from build123d import *

# Parameters (mm, degrees)
SKETCH1_R           = 2
BOSS_EXTRUDE1_DEPTH = 2.5
SKETCH2_W           = 35
SKETCH2_H           = 4
BOSS_EXTRUDE2_DEPTH = 35
CUT_EXTRUDE1_REACH  = 6
SKETCH3_R           = 1.5
SKETCH3_R_2         = 7.75


with BuildPart() as part:
    # Sketch1 → Boss-Extrude1 (new body, symmetric)
    with BuildSketch(Plane(origin=(0, 0, 0), x_dir=(1, 0, 0), z_dir=(0, 1, 0))):
        Polygon((17.5, 45), (-5.5, 45), (-5.5, -10), (-17.5, -10), (-17.5, -45), (17.5, -45), align=None)
        with Locations((-11.75, -20)):
            Circle(SKETCH1_R, mode=Mode.SUBTRACT)
        with BuildLine():
            ThreePointArc((13.75, -20), (11.75, -22), (9.75, -20))
            ThreePointArc((9.75, -20), (11.75, -18), (13.75, -20))
        make_face(mode=Mode.SUBTRACT)
        with Locations((11.75, -1.5)):
            Circle(SKETCH1_R, mode=Mode.SUBTRACT)
    extrude(amount=BOSS_EXTRUDE1_DEPTH, both=True)

    # Sketch2 → Boss-Extrude2 (add)
    with BuildSketch(Plane(origin=(0, 2.5, 0), x_dir=(1, 0, 0), z_dir=(0, 1, 0))):
        with Locations((0, -43)):
            Rectangle(SKETCH2_W, SKETCH2_H)
    extrude(amount=BOSS_EXTRUDE2_DEPTH)

    # Sketch3 → Cut-Extrude1 (cut, up to next)
    with BuildSketch(Plane(origin=(0, 0, 41), x_dir=(-1, 0, 0), z_dir=(0, 0, -1)), mode=Mode.PRIVATE) as cut_extrude1_sk1:
        with Locations((-12.2, 20)):
            Circle(SKETCH3_R)
    cut_extrude1_tool1 = extrude(cut_extrude1_sk1.sketch, amount=-CUT_EXTRUDE1_REACH, mode=Mode.PRIVATE) & part.part
    add(cut_extrude1_tool1.solids().sort_by_distance((12.2, 20, 41))[0], mode=Mode.SUBTRACT)
    # Sketch3 → Cut-Extrude1 (cut, up to next)
    with BuildSketch(Plane(origin=(0, 0, 41), x_dir=(-1, 0, 0), z_dir=(0, 0, -1)), mode=Mode.PRIVATE) as cut_extrude1_sk2:
        with Locations((0, 32.2)):
            Circle(SKETCH3_R)
    cut_extrude1_tool2 = extrude(cut_extrude1_sk2.sketch, amount=-CUT_EXTRUDE1_REACH, mode=Mode.PRIVATE) & part.part
    add(cut_extrude1_tool2.solids().sort_by_distance((0, 32.2, 41))[0], mode=Mode.SUBTRACT)
    # Sketch3 → Cut-Extrude1 (cut, up to next)
    with BuildSketch(Plane(origin=(0, 0, 41), x_dir=(-1, 0, 0), z_dir=(0, 0, -1)), mode=Mode.PRIVATE) as cut_extrude1_sk3:
        with Locations((12.2, 20)):
            Circle(SKETCH3_R)
    cut_extrude1_tool3 = extrude(cut_extrude1_sk3.sketch, amount=-CUT_EXTRUDE1_REACH, mode=Mode.PRIVATE) & part.part
    add(cut_extrude1_tool3.solids().sort_by_distance((-12.2, 20, 41))[0], mode=Mode.SUBTRACT)
    # Sketch3 → Cut-Extrude1 (cut, up to next)
    with BuildSketch(Plane(origin=(0, 0, 41), x_dir=(-1, 0, 0), z_dir=(0, 0, -1)), mode=Mode.PRIVATE) as cut_extrude1_sk4:
        with Locations((0, 20)):
            Circle(SKETCH3_R_2)
    cut_extrude1_tool4 = extrude(cut_extrude1_sk4.sketch, amount=-CUT_EXTRUDE1_REACH, mode=Mode.PRIVATE) & part.part
    add(cut_extrude1_tool4.solids().sort_by_distance((0, 20, 41))[0], mode=Mode.SUBTRACT)
    # Sketch3 → Cut-Extrude1 (cut, up to next)
    with BuildSketch(Plane(origin=(0, 0, 41), x_dir=(-1, 0, 0), z_dir=(0, 0, -1)), mode=Mode.PRIVATE) as cut_extrude1_sk5:
        with Locations((0, 7.8)):
            Circle(SKETCH3_R)
    cut_extrude1_tool5 = extrude(cut_extrude1_sk5.sketch, amount=-CUT_EXTRUDE1_REACH, mode=Mode.PRIVATE) & part.part
    add(cut_extrude1_tool5.solids().sort_by_distance((0, 7.8, 41))[0], mode=Mode.SUBTRACT)


solid = part.part
Work out the finished part from the listing and answer in its coordinate system (mm). A direction names the side the tool comes from. Give positions to 0.01 mm unless a question says otherwise; leave off trailing zeros. Loops run counter-clockwise (first coordinate to the right, second up) from the corner with the lowest first, then second, coordinate; pieces in that order, holes last. Notation, with made-up numbers: (14, 22) -> (63, 22) arc R24 cw to (63, 34) -> close; hole circle Ø5 at (8, 72.25). An arc over 180 degrees is marked (long way). Use a Markdown table: item, result. Add a question column.
1) Which of the six approach directions +Z, -Z, +X, -X, +Y, -Y give full straight-line access (tool end or side, diameter ignored) to faces 1 (the flat face through (-11, 0, 10)), 2 (the flat face through (4, 2.5, -3)), 3 (the flat face through (17.5, 1, 10))?
2) The part is cut by section B-B, the plane y = 7.8. Determine the outline of the cut face in (x, z).
3) Consider line 1 along Y through (x, z) = (0, 42); line 2 along X through (y, z) = (-1, 20); line 3 along Z through (x, y) = (11.75, 0.5). Determine where each line is inside the solid, lowest interval first.
4) The part is cut by section D-D, the plane x = 4. Determine the outline of the cut face in (y, z), plus the area to 3 significant figures.
5) Each of these flat-tipped pins is pushed along its axis until it touches: P1, Ø3, axis at x = -4.5, z = 21, coming from the +Y side; P2, Ø2, axis at y = 4.5, z = -6.5, coming from the +X side; P3, Ø4, axis at x = 0, y = 7.8, coming from the -Z side; P4, Ø1.5, axis at y = 1, z = -13, coming from the -X side. Where does it stop, or does it pass through?
6) The part is cut by section A-A, the plane z = 20. Determine the outline of the cut face in (x, y), plus the area to 3 significant figures.
7) For a pull along Y with two mould halves and no side action, classify faces 4 (the cylindrical face through (1.009, 27.684, 42.972)), 5 (the flat face through (4, -2.5, -1)), 6 (the flat face through (0, 37.5, 43)) as +Y half, -Y half, draft (parallel to the pull), parting line (faces both ways), or undercut.
8) The part is cut by section C-C, the plane z = 1.5. Determine the outline of the cut face in (x, y).
Reported:
| question | item | result |
|---|---|---|
| 1 | face 1 | -Z, -X, +Y, -Y |
| 1 | face 2 | -Z, +X, -X, +Y |
| 1 | face 3 | +Z, -Z, +X, +Y, -Y |
| 2 | outline | (-17.5, 41) -> (-1.5, 41) -> (-1.5, 45) -> (-17.5, 45) -> close; (1.5, 41) -> (17.5, 41) -> (17.5, 45) -> (1.5, 45) -> close |
| 3 | line 1 | y = -2.5 to 6.3, 9.3 to 12.25, 27.75 to 30.7, 33.7 to 37.5 |
| 3 | line 2 | x = -17.5 to -13.75, -9.75 to 9.75, 13.75 to 17.5 |
| 3 | line 3 | z = -45 to -0.5, 3.5 to 18, 22 to 45 |
| 4 | outline | (-2.5, -45) -> (2.5, -45) -> (2.5, 41) -> (13.36, 41) -> (13.36, 45) -> (-2.5, 45) -> close; (26.64, 41) -> (37.5, 41) -> (37.5, 45) -> (26.64, 45) -> close |
| 4 | area | 537 mm^2 |
| 5 | P1 | stops at y = 2.5 |
| 5 | P2 | passes through |
| 5 | P3 | stops at z = 41 |
| 5 | P4 | stops at x = -5.5 |
| 6 | outline | (-17.5, -2.5) -> (-13.75, -2.5) -> (-13.75, 2.5) -> (-17.5, 2.5) -> close; (-9.75, -2.5) -> (9.75, -2.5) -> (9.75, 2.5) -> (-9.75, 2.5) -> close; (13.75, -2.5) -> (17.5, -2.5) -> (17.5, 2.5) -> (13.75, 2.5) -> close |
| 6 | area | 135 mm^2 |
| 7 | face 4 | undercut |
| 7 | face 5 | -Y half |
| 7 | face 6 | +Y half |
| 8 | outline | (-5.5, -2.5) -> (9.75, -2.5) -> (9.75, 2.5) -> (-5.5, 2.5) -> close; (13.75, -2.5) -> (17.5, -2.5) -> (17.5, 2.5) -> (13.75, 2.5) -> close |
